from build123d import *

# Parameters (mm, degrees)
F0_W     = 19.6
F0_H     = 33.2
F1_DEPTH = 40
F2_DEPTH = 10
F3_DEPTH = 2


# Not quite as in the source:
# - a feature names something its author has since deleted; it is built from what else it names


with BuildPart() as f1:
    # F0 (on Top) → F1 (new body)
    with BuildSketch(Plane.XY):
        Polygon((0, 0), (0, -3.6), (2.9, -3.6), (26, -3.6), (26, 0), (26, 36.4), (0, 36.4), align=None)
        with Locations((13, 16.6)):
            Rectangle(F0_W, F0_H, mode=Mode.SUBTRACT)
    extrude(amount=F1_DEPTH)

    # F0 (on Top) → F2 (join)
    with BuildSketch(Plane.XY):
        Polygon((86.8, -90), (90, -90), (90, -87.4), (90, 0), (26, 0), (26, -3.6), (86.8, -3.6), (86.8, -87.4), (2.9, -87.4), (2.9, -3.6), (0, -3.6), (0, -90), align=None)
    extrude(amount=F2_DEPTH)

    # F0 (on Top) → F3 (join)
    with BuildSketch(Plane.XY):
        with Locations((13, 16.6)):
            Rectangle(F0_W, F0_H)
    extrude(amount=F3_DEPTH)


solid = f1.part
CAD build for the part. Positions are in the model's coordinates, mm. A direction names the side the tool comes from. Round coordinates to 2 decimals unless told otherwise and drop trailing zeros. Write each loop counter-clockwise with the first axis right and the second up, starting at its lowest first coordinate (ties: lowest second). Pieces come first, ordered by that corner, then holes.
(1) Slice it at C-C, the plane z = 5.5. Write the cut outline in (x, y), and give its area (3 significant figures).
(2) Slice it at B-B, the plane x = 36. Write the cut outline in (y, z), and give its area (3 significant figures).
(3) 3-axis set-ups, long thin cutter, end or side, ignore diameter. For faces 5 (the face through (48, -88, 10)), 6 (the face through (13, 0, 21)), 7 (the face through (86.8, -45, 5)): which of +Z, -Z, +X, -X, +Y, -Y reach the whole face in a straight line?
(4) Drop flat-ended pins along their axis: P1, Ø3, axis at x = 43, z = 5, coming from the +Y side; P2, Ø6, axis at x = 12, z = 29.5, coming from the -Y side; P3, Ø10, axis at x = 15, y = 20, coming from the +Z side. Give the stop position or say it passes through.
(5) Mould opens along Y. For faces 1 (the face through (13, 33.2, 21)), 2 (the face through (1, 17, 40)), 3 (the face through (44, -90, 5)), 4 (the face through (58, 0, 5)) say: pulls with the +Y half, pulls with the -Y half, needs draft (parallel to the pull), parting line crosses it, or undercut.
(6) Slice it at A-A, the plane y = -29.5. Write the cut outline in (x, z).
(7) Slice it at D-D, the plane z = 37. Write the cut outline in (x, y), and give its area (3 significant figures).
(8) Probe line 1 along Y through (x, z) = (19.5, 7); line 2 along X through (y, z) = (7.5, 30.5); line 3 along X through (y, z) = (-64.5, 4). List the from-to ranges inside material, lowest first.
From the geometry:
1. outline: (0, -90) - (90, -90) - (90, 0) - (26, 0) - (26, 36.4) - (0, 36.4) - close; hole (2.9, -87.4) - (86.8, -87.4) - (86.8, -3.6) - (2.9, -3.6) - close; hole (3.2, 0) - (22.8, 0) - (22.8, 33.2) - (3.2, 33.2) - close
1. area: 1,360 mm2
2. outline: (-90, 0) - (-87.4, 0) - (-87.4, 10) - (-90, 10) - close; (-3.6, 0) - (0, 0) - (0, 10) - (-3.6, 10) - close
2. area: 62.0 mm2
3. face 5: +Z, +X, -Y
3. face 6: +Z
3. face 7: +Z, -Z
4. P1: stops at y = 0
4. P2: stops at y = -3.6
4. P3: stops at z = 2
5. face 1: undercut
5. face 2: needs draft
5. face 3: pulls with the -Y half
5. face 4: pulls with the +Y half
6. outline: (0, 0) - (2.9, 0) - (2.9, 10) - (0, 10) - close; (86.8, 0) - (90, 0) - (90, 10) - (86.8, 10) - close
7. outline: (0, -3.6) - (26, -3.6) - (26, 36.4) - (0, 36.4) - close; hole (3.2, 0) - (22.8, 0) - (22.8, 33.2) - (3.2, 33.2) - close
7. area: 389 mm2
8. line 1: y = -90 to -87.4, -3.6 to 0, 33.2 to 36.4
8. line 2: x = 0 to 3.2, 22.8 to 26
8. line 3: x = 0 to 2.9, 86.8 to 90
